Autodesk Inventor part; units mm, degrees
ref_plane "YZ Plane" through (0, 0, 0) normal (1, 0, 0) x (0, 1, 0)
ref_plane "XZ Plane" through (0, 0, 0) normal (0, 1, 0) x (-1, 0, 0)
ref_plane "XY Plane" through (0, 0, 0) normal (0, 0, 1) x (1, 0, 0)
ref_plane "РабПлоскость1" through (0, 0, 0) normal (0, 0, 1) x (1, 0, 0)
sketch "Эскиз1" plane through (0, 0, 0) normal (0, 0, 1) x (1, 0, 0)
  line L0 (36.1495, -96.5) -> (-43.8505, -96.5)
  line L1 (-43.8505, -96.5) -> (-43.8505, -106.5)
  line L2 (-43.8505, -106.5) -> (36.1495, -106.5)
  line L3 (36.1495, -106.5) -> (36.1495, -96.5)
  line L4 (22.5, -91.5) -> (-22.5, -91.5)
  circle A0 centre (0, -101.5) radius 2
  circle A1 centre (22.5, -101.5) radius 2
  circle A2 centre (-22.5, -101.5) radius 2
  point P0 (0, 0)
  dimension "d0" = 80
  dimension "d1" = 10
  dimension "d2" = 5
  dimension "d3" = 4
  dimension "d5" = 4
  dimension "d6" = 4
extrude "Выдавливание1" add sketch "Эскиз1" along normal blind 2
sketch "Эскиз2" plane through (0, 0, 2) normal (0, 0, 1) x (1, 0, 0)
  point P0 (0, 0)
sketch "Эскиз3" plane through (-43.8505, -106.5, 0) normal (0, -1, 0) x (1, 0, 0)
  line L0 (0, 0) -> (0, 2)
  line L1 (0, 2) -> (0, 13.9799)
  line L2 (0, 13.9799) -> (7, 13.9799)
  line L3 (7, 13.9799) -> (7, 9)
  line L4 (7, 9) -> (73, 9)
  line L5 (73, 9) -> (73, 13.9799)
  line L6 (73, 13.9799) -> (80, 13.9799)
  line L7 (80, 13.9799) -> (80, 2)
  line L8 (0, 2) -> (80, 2)
  point P0 (43.8505, 0)
  point P1 (80, 2)
  dimension "d9" = 7
  dimension "d10" = 7
  dimension "d15" = 7
extrude "Выдавливание2" add sketch "Эскиз3" against normal blind 2
sketch "Эскиз4" plane through (-43.8505, -96.5, 0) normal (0, 1, 0) x (1, 0, 0)
  line L0 (0, -2) -> (80, -2)
  line L1 (0, -2) -> (0, -13.9799)
  line L2 (0, -13.9799) -> (7, -13.9799)
  line L3 (7, -13.9799) -> (7, -9)
  line L4 (7, -9) -> (73, -9)
  line L5 (73, -9) -> (73, -13.9799)
  line L6 (73, -13.9799) -> (80, -13.9799)
  line L7 (80, -13.9799) -> (80, -2)
  point P0 (43.8505, 0)
extrude "Выдавливание3" add sketch "Эскиз4" against normal blind 2
sketch "Эскиз5" plane through (-36.8505, -96.5, 9) normal (0, 0, 1) x (1, 0, 0)
  line L0 (66, -10) -> (0, -10)
  line L1 (3.8262, -0.07) -> (63.012, -0.07)
  line L2 (63.012, -10) -> (3.8262, -10)
  line L3 (66, 0) -> (66, -2)
  line L4 (0, -10) -> (66, -10)
  line L5 (66, -10) -> (66, 0)
  line L6 (66, 0) -> (0, 0)
  line L7 (0, 0) -> (0, -10)
  point P0 (36.8505, 96.5)
extrude "Выдавливание4" add sketch "Эскиз5" along normal blind 2
properties part number "деталь держит провода"
Work out the finished part from the listing and answer in its coordinate system (mm). A direction names the side the tool comes from. Round coordinates to 2 decimals unless told otherwise and drop trailing zeros. Loops run counter-clockwise (first coordinate to the right, second up) from the corner with the lowest first, then second, coordinate; pieces in that order, holes last. Notation, with made-up numbers: (70, -29) - (82, -29) arc R27 ccw to (82, 5) - close; hole circle Ø5 at (-14.75, 45.25). An arc over 180 degrees is marked (long way). Use one line per item in the form item = value. Start each with the question number.
(1) Find section B-B on y = -101.5. Determine the outline of the cut face in (x, z), and give its area (3 significant figures).
(2) Consider line 1 (Y direction, x = -22.5, z = 0.7); line 2 (Y direction, x = -3.5, z = 8.5); line 3 (Z direction, x = -29, y = -100.5). Determine where each line is inside the solid, lowest interval first.
(3) Find section D-D on z = 7.5. Determine the outline of the cut face in (x, y), and give its area (3 significant figures).
(4) Find section A-A on z = 11.75. Determine the outline of the cut face in (x, y).
(5) Find section C-C on x = 22.5. Determine the outline of the cut face in (y, z), and give its area (3 significant figures).
(6) Which of the six approach directions +Z, -Z, +X, -X, +Y, -Y give full straight-line access (tool end or side, diameter ignored) to faces 5 (the face through (-36.85, -101, 10)), 6 (the face through (-22.76, -103.483, 0.986)), 7 (the face through (-4, -101, 2)), 8 (the face through (29.15, -102, 10)), 9 (the face through (-4, -101, 11))?
(7) Flat-ended cylindrical pins translate along their axes: P1, Ø2, axis at y = -101.5, z = 10, coming from the -X side; P2, Ø3, axis at x = -10.5, y = -102, coming from the +Z side; P3, Ø3, axis at y = -102, z = 11, coming from the +X side. Find the tip coordinate at first contact, or state that the pin passes through.
(8) Determine the mould class of faces 1 (the face through (-36.85, -106, 13)), 2 (the face through (-36.85, -97, 13)), 3 (the face through (-40, -106, 13.98)), 4 (the face through (36.15, -105, 7)) for opening direction X: +X half, -X half, draft (parallel to the pull), parting line (faces both ways), or undercut.
Answer list:
q1.outline = (-43.85, 0) - (-24.5, 0) - (-24.5, 2) - (-43.85, 2) - close; (-36.85, 9) - (29.15, 9) - (29.15, 11) - (-36.85, 11) - close; (-20.5, 0) - (-2, 0) - (-2, 2) - (-20.5, 2) - close; (2, 0) - (20.5, 0) - (20.5, 2) - (2, 2) - close; (24.5, 0) - (36.15, 0) - (36.15, 2) - (24.5, 2) - close
q1.area = 268 mm^2
q2.line_1 = -106.5 to -103.5, -99.5 to -96.5
q2.line_2 = -106.5 to -104.5, -98.5 to -96.5
q2.line_3 = 0 to 2, 9 to 11
q3.outline = (-43.85, -106.5) - (36.15, -106.5) - (36.15, -104.5) - (-43.85, -104.5) - close; (-43.85, -98.5) - (36.15, -98.5) - (36.15, -96.5) - (-43.85, -96.5) - close
q3.area = 320 mm^2
q4.outline = (-43.85, -106.5) - (-36.85, -106.5) - (-36.85, -104.5) - (-43.85, -104.5) - close; (-43.85, -98.5) - (-36.85, -98.5) - (-36.85, -96.5) - (-43.85, -96.5) - close; (29.15, -106.5) - (36.15, -106.5) - (36.15, -104.5) - (29.15, -104.5) - close; (29.15, -98.5) - (36.15, -98.5) - (36.15, -96.5) - (29.15, -96.5) - close
q5.outline = (-106.5, 0) - (-103.5, 0) - (-103.5, 2) - (-104.5, 2) - (-104.5, 9) - (-98.5, 9) - (-98.5, 2) - (-99.5, 2) - (-99.5, 0) - (-96.5, 0) - (-96.5, 11) - (-106.5, 11) - close
q5.area = 60.0 mm^2
q6.face_5 = +Z, -X
q6.face_6 = -Z
q6.face_7 = +X, -X
q6.face_8 = +Z, +X
q6.face_9 = +Z, +Y, -Y
q7.P1 = -36.85
q7.P2 = 11
q7.P3 = 29.15
q8.face_1 = undercut
q8.face_2 = undercut
q8.face_3 = draft
q8.face_4 = +X half
